The listing builds one solid part. Answer for the finished solid, in the listing's coordinates (mm). Coordinates: 2 decimals unless noted, no trailing zeros. Order: outer loops, then holes, each group sorted by start corner. A loop starts at its lowest first (then second) coordinate and runs counter-clockwise, first axis right, second up. Notation, with made-up numbers: (-24, -36) -> (-4, -36) arc R16 ccw to (-4, -25) -> close; hole circle Ø9 at (2.5, -2.75). An arc over 180 degrees is marked (long way). Answer in a Markdown table with one row per item.
```python
from build123d import *

# Parameters (mm, degrees)
F0_R     = 5
F1_DEPTH = 8
F3_DEPTH = 24
F4_DEPTH = 20
F5_D     = 10
F5_DEPTH = 24
F5_TIP   = 3.0043030951


with BuildPart() as f1:
    # F0 (on Top) → F1 (new body)
    with BuildSketch(Plane.XY):
        with BuildLine():
            Line((19, 0), (0, 0))
            Line((0, 0), (-19, 0))
            ThreePointArc((-19, 0), (-29, -10), (-19, -20))
            Line((-19, -20), (0, -20))
            Line((0, -20), (19, -20))
            ThreePointArc((19, -20), (29, -10), (19, 0))
        make_face()
        with Locations((-19, -10)):
            Circle(F0_R, mode=Mode.SUBTRACT)
        with Locations((19, -10)):
            Circle(F0_R, mode=Mode.SUBTRACT)
    extrude(amount=F1_DEPTH)

    # F2 (on face) → F3 (join)
    with BuildSketch(Plane(origin=(0, 0, 0), x_dir=(-1, 0, 0), z_dir=(0, 1, 0))):
        with BuildLine():
            ThreePointArc((4, 8), (0, 6), (-4, 8))
            Line((-4, 8), (-6.3245553203, 8))
            ThreePointArc((-6.3245553203, 8), (0, 4), (6.3245553203, 8))
            Line((6.3245553203, 8), (4, 8))
        make_face()
        with BuildLine():
            ThreePointArc((-4, 8), (-1.5811388301, 15.7434164903), (5, 11))
            ThreePointArc((5, 11), (4.7434164903, 9.4188611699), (4, 8))
            Line((4, 8), (6.3245553203, 8))
            ThreePointArc((6.3245553203, 8), (6.8290514437, 9.4624511784), (7, 11))
            ThreePointArc((7, 11), (-1.5375488216, 17.8290514437), (-6.3245553203, 8))
            Line((-6.3245553203, 8), (-4, 8))
        make_face()
    extrude(amount=-F3_DEPTH)

    # F2 (on face) → F4 (join)
    with BuildSketch(Plane(origin=(0, 0, 0), x_dir=(-1, 0, 0), z_dir=(0, 1, 0))):
        with BuildLine():
            Line((-9.5393920142, 8), (-6.3245553203, 8))
            ThreePointArc((-6.3245553203, 8), (-1.5375488216, 17.8290514437), (7, 11))
            ThreePointArc((7, 11), (6.8290514437, 9.4624511784), (6.3245553203, 8))
            Line((6.3245553203, 8), (9.5393920142, 8))
            ThreePointArc((9.5393920142, 8), (9.8841772582, 9.4824230072), (10, 11))
            ThreePointArc((10, 11), (0, 21), (-10, 11))
            ThreePointArc((-10, 11), (-9.8841772582, 9.4824230072), (-9.5393920142, 8))
        make_face()
    extrude(amount=-F4_DEPTH)

    # F5
    with Locations(Plane(origin=(0, 0, 0), x_dir=(-1, 0, 0), z_dir=(0, 1, 0))):
        with Locations((0, 11)):
            Hole(F5_D / 2, depth=F5_DEPTH)
            with Locations((0, 0, -(F5_DEPTH + F5_TIP / 2))):  # 118° drill point
                Cone(0, F5_D / 2, F5_TIP, mode=Mode.SUBTRACT)


solid = f1.part
```
(1) A cutting plane is placed at C-C, the plane x = 0. Determine the outline of the cut face in (y, z).
Check values:
| item | result |
|---|---|
| outline | (-24, 4) -> (-20, 4) -> (-20, 0) -> (0, 0) -> (0, 6) -> (-24, 6) -> close; (-24, 16) -> (0, 16) -> (0, 21) -> (-20, 21) -> (-20, 18) -> (-24, 18) -> close |
(2) A cutting plane is placed at D-D, the plane y = -21. Determine the outline of the cut face in (x, z).
Check values:
| item | result |
|---|---|
| outline | circle Ø14 at (0, 11); hole circle Ø10 at (0, 11) |
(3) Find the intervals of material crossed by line 1 along Y through (x, z) = (-19, 6.75); line 2 along X through (y, z) = (-6.5, 3.25); line 3 along Y through (x, z) = (8, 14.5), in increasing order. Write a range as from..to.
Check values:
| item | result |
|---|---|
| line 1 | -20..-15, -5..0 |
| line 2 | -28.37..-22.57, -15.43..15.43, 22.57..28.37 |
| line 3 | -20..0 |
(4) For a pull along X with two mould halves and no side action, classify faces 1 (the flat face through (5, -24, 13)), 2 (the cylindrical face through (18.349, -5.043, 3.944)), 3 (the cylindrical face through (-23, -7, 4)), 4 (the cylindrical face through (29, -10, 4)) as released by +X, released by -X, zero draft, split by the parting line, or undercut.
Check values:
| item | result |
|---|---|
| face 1 | zero draft |
| face 2 | undercut |
| face 3 | undercut |
| face 4 | released by +X |
(5) A cutting plane is placed at B-B, the plane z = 14. Determine the outline of the cut face in (x, y).
Check values:
| item | result |
|---|---|
| outline | (-9.54, -20) -> (-6.32, -20) -> (-6.32, -24) -> (-4, -24) -> (-4, 0) -> (-9.54, 0) -> close; (4, -24) -> (6.32, -24) -> (6.32, -20) -> (9.54, -20) -> (9.54, 0) -> (4, 0) -> close |
(6) A cutting plane is placed at A-A, the plane y = -10. Determine the outline of the cut face in (x, z).
Check values:
| item | result |
|---|---|
| outline | (-29, 0) -> (-24, 0) -> (-24, 8) -> (-29, 8) -> close; (-14, 0) -> (14, 0) -> (14, 8) -> (9.54, 8) arc R10 ccw (long way) to (-9.54, 8) -> (-14, 8) -> close; (24, 0) -> (29, 0) -> (29, 8) -> (24, 8) -> close; hole circle Ø10 at (0, 11) |
(7) Flat-ended cylindrical pins translate along their axes: pin 1 (6 mm diameter, centred on y = -14, z = 8, fed in from -X); pin 2 (3 mm diameter, centred on x = -6, y = -10, fed in from +Z); pin 3 (1 mm diameter, centred on x = 8.5, y = -4, fed in from +Z); pin 4 (3 mm diameter, centred on x = 20, y = -21.5, fed in from +Z). Find the tip coordinate at first contact, or state that the pin passes through.
Check values:
| item | result |
|---|---|
| pin 1 | x = -28.95 |
| pin 2 | z = 19.93 |
| pin 3 | z = 17 |
| pin 4 | through |
